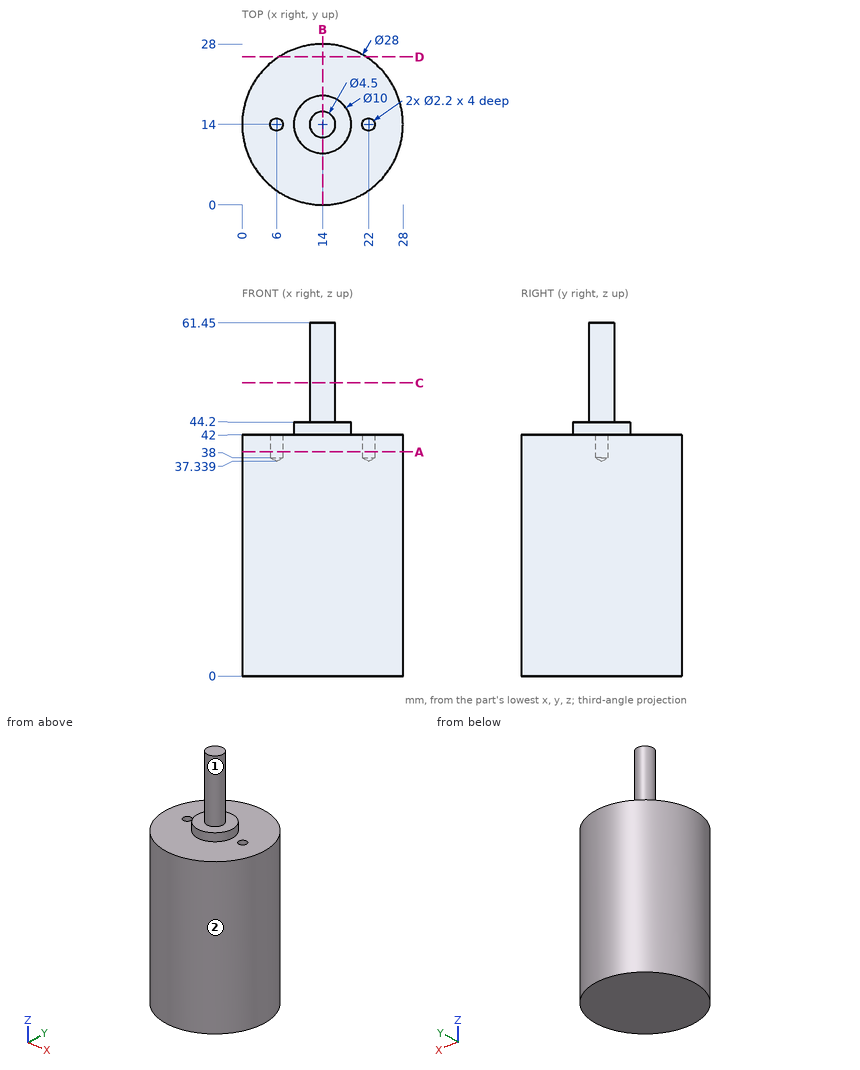
The figure shows three views and two pictorial views of one solid part (mm, origin at its lowest corner). Answer the questions. A direction names the side the tool comes from. Round coordinates to 2 decimals unless told otherwise and drop trailing zeros. Loops run counter-clockwise (first coordinate to the right, second up) from the corner with the lowest first, then second, coordinate; pieces in that order, holes last. Notation, with made-up numbers: (16.5, 38) - (49.5, 38) arc R13 ccw to (49.5, 51) - close; hole circle Ø3 at (38, -34.75). An arc over 180 degrees is marked (long way). Use one line per item in the form item = value. Start each with the question number.
(1) Consider line 1 (Z direction, x = 11, y = 13.25); line 2 (Z direction, x = 23, y = 21.25); line 3 (Y direction, x = 22, z = 40.7). Determine where each line is inside the solid, lowest interval first.
(2) Flat-ended cylindrical pins translate along their axes: P1, Ø2, axis at x = 23, z = 21.5, coming from the -Y side; P2, Ø2, axis at y = 11, z = 11, coming from the -X side; P3, Ø4, axis at x = 10, z = 18, coming from the +Y side. Find the tip coordinate at first contact, or state that the pin passes through.
(3) Find section C-C on z = 51. Determine the outline of the cut face in (x, y), and give its area (3 significant figures).
(4) Find section B-B on x = 14. Determine the outline of the cut face in (y, z).
(5) Which of the six approach directions +Z, -Z, +X, -X, +Y, -Y give full straight-line access (tool end or side, diameter ignored) to the marked faces 1 and 2?
(6) Find section D-D on y = 25.75. Determine the outline of the cut face in (x, z), and give its area (3 significant figures).
(7) Find section A-A on z = 39. Determine the outline of the cut face in (x, y), and give its area (3 significant figures).
Answer list:
q1.line_1 = 0 to 44.2
q1.line_2 = 0 to 42
q1.line_3 = 2.51 to 12.9, 15.1 to 25.49
q2.P1 = 2.51
q2.P2 = 0.14
q2.P3 = 27.86
q3.outline = circle Ø4.5 at (14, 14)
q3.area = 15.9 mm^2
q4.outline = (0, 0) - (28, 0) - (28, 42) - (19, 42) - (19, 44.2) - (16.25, 44.2) - (16.25, 61.45) - (11.75, 61.45) - (11.75, 44.2) - (9, 44.2) - (9, 42) - (0, 42) - close
q5.face_1 = +Z
q5.face_2 = +Z, -Z
q6.outline = (6.39, 0) - (21.61, 0) - (21.61, 42) - (6.39, 42) - close
q6.area = 639 mm^2
q7.outline = circle Ø28 at (14, 14); hole circle Ø2.2 at (6, 14); hole circle Ø2.2 at (22, 14)
q7.area = 608 mm^2
